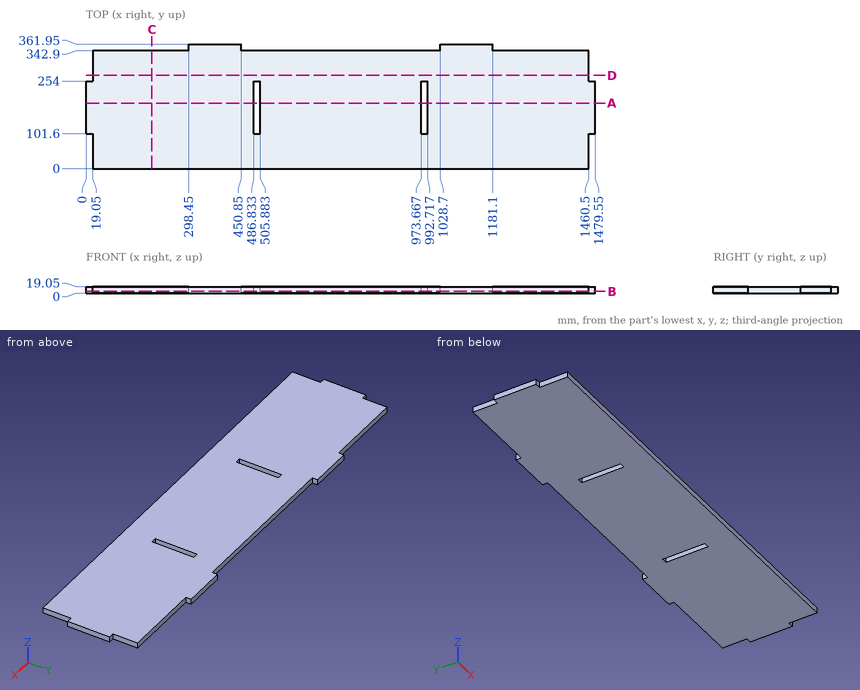
Drawing for the job (mm, zero at the part's lowest x, y, z). Give positions to 0.01 mm unless a question says otherwise; leave off trailing zeros. Loops run counter-clockwise (first coordinate to the right, second up) from the corner with the lowest first, then second, coordinate; pieces in that order, holes last. Notation, with made-up numbers: (40.5, 61) - (70.5, 61) arc R22 cw to (70.5, 78) - close; hole circle Ø10 at (14.5, 34). An arc over 180 degrees is marked (long way). Write item = value, one per line. Start each with the question number.
1) Band-saw the part on C-C on x = 191. Give the cut face in (y, z).
2) Band-saw the part on D-D on y = 271. Give the cut face in (x, z), plus the area to 3 significant figures.
3) Probe probe 1 along X at (y, z) = (151.5, 13.5); probe 2 along X at (y, z) = (97, 17); probe 3 along Y at (x, z) = (915, 14). List the from-to ranges inside material, lowest first. Write a range as from..to.
4) Band-saw the part on A-A on y = 190. Give the cut face in (x, z).
5) Drop flat-ended pins along their axis: pin 1 Ø12 at (x, y) = (1279, 66.5) entering from -Z; pin 2 Ø9.5 at (y, z) = (350.5, 13.5) entering from +X; pin 3 Ø5.5 at (x, z) = (495.5, 6.5) entering from +Y; pin 4 Ø9.5 at (x, z) = (5.5, 9.5) entering from -Y. Give the stop position or say it passes through.
6) Band-saw the part on B-B on z = 5. Give the cut face in (x, y), plus the area to 3 significant figures.
Final values:
q1.outline = (0, 0) - (342.9, 0) - (342.9, 19.05) - (0, 19.05) - close
q2.outline = (19.05, 0) - (1460.5, 0) - (1460.5, 19.05) - (19.05, 19.05) - close
q2.area = 27,500 mm²
q3.probe_1 = 0..486.83, 505.88..973.67, 992.72..1479.55
q3.probe_2 = 19.05..1460.5
q3.probe_3 = 0..342.9
q4.outline = (0, 0) - (486.83, 0) - (486.83, 19.05) - (0, 19.05) - close; (505.88, 0) - (973.67, 0) - (973.67, 19.05) - (505.88, 19.05) - close; (992.72, 0) - (1479.55, 0) - (1479.55, 19.05) - (992.72, 19.05) - close
q5.pin_1 = 0
q5.pin_2 = 1181.1
q5.pin_3 = 342.9
q5.pin_4 = 101.6
q6.outline = (0, 101.6) - (19.05, 101.6) - (19.05, 0) - (1460.5, 0) - (1460.5, 101.6) - (1479.55, 101.6) - (1479.55, 254) - (1460.5, 254) - (1460.5, 342.9) - (1181.1, 342.9) - (1181.1, 361.95) - (1028.7, 361.95) - (1028.7, 342.9) - (450.85, 342.9) - (450.85, 361.95) - (298.45, 361.95) - (298.45, 342.9) - (19.05, 342.9) - (19.05, 254) - (0, 254) - close; hole (486.83, 101.6) - (505.88, 101.6) - (505.88, 254) - (486.83, 254) - close; hole (973.67, 101.6) - (992.72, 101.6) - (992.72, 254) - (973.67, 254) - close
q6.area = 500,000 mm²
